Build history of the part. All positions in model axes, mm. Face numbers are marked on the shaded views. A direction names the side the tool comes from. Give positions to 0.01 mm unless a question says otherwise; leave off trailing zeros. Loops run counter-clockwise (first coordinate to the right, second up) from the corner with the lowest first, then second, coordinate; pieces in that order, holes last. Notation, with made-up numbers: (58, 81) -> (102, 81) arc R15 ccw to (102, 86) -> close; hole circle Ø10 at (8.5, 45). An arc over 180 degrees is marked (long way). Answer as a JSON object with one key per item and string values. Group by question number.
Q1. Band-saw the part on A-A, the plane y = 7.75. Write the cut outline in (x, z), plus the area to 3 significant figures.
Q2. Band-saw the part on B-B, the plane x = 16.25. Write the cut outline in (y, z), plus the area to 3 significant figures.
Q3. Band-saw the part on D-D, the plane z = 2.2. Write the cut outline in (x, y), plus the area to 3 significant figures.
Q4. Wall check: probe 1 along X at (y, z) = (15.75, 3.25); probe 2 along Y at (x, z) = (12, 1.85); probe 3 along X at (y, z) = (17.5, 0.4). Give the ranges that are in metal, low to high. Write a range as from..to.
Q5. Tool access for the marked faces 1 and 2: list every direction of +Z, -Z, +X, -X, +Y, -Y with a clear straight run to the whole face (end or side of a thin tool).
Q6. Band-saw the part on C-C, the plane y = 15.5. Write the cut outline in (x, z).
Q7. Drop flat-ended pins along their axis: pin 1 (5 mm diameter, centred on x = 15.52, y = 15.79, fed in from +Z); pin 2 (4 mm diameter, centred on x = 5.77, y = 15.79, fed in from +Z). Give the stop position or say it passes through.
Q8. Two-plate mould, pull along X, no slides. Class the marked faces 3, 4, 5 and 6: pulls with the +X half, pulls with the -X half, needs draft (parallel to the pull), parting line crosses it, or undercut.
from build123d import *

# Parameters (mm, degrees)
ESQUISSE1_W        = 21.281999849
ESQUISSE1_H        = 19.97412287
ESQUISSE1_R        = 2.13
ESQUISSE1_W_2      = 4
ESQUISSE1_H_2      = 7
BOSS_EXTRU_1_DEPTH = 4
CONG_1_R           = 2


with BuildPart() as part:
    # Esquisse1 → Boss.-Extru.1 (new body)
    with BuildSketch(Plane.XY):
        with Locations((10.640999925, 9.987061435)):
            Rectangle(ESQUISSE1_W, ESQUISSE1_H)
        with Locations((5.765999924, 15.79412287)):
            Circle(ESQUISSE1_R, mode=Mode.SUBTRACT)
        with Locations((15.515999924, 15.79412287)):
            Circle(ESQUISSE1_R, mode=Mode.SUBTRACT)
        with Locations((10.640999924, 5.79412287)):
            Rectangle(ESQUISSE1_W_2, ESQUISSE1_H_2, mode=Mode.SUBTRACT)
    extrude(amount=BOSS_EXTRU_1_DEPTH)

    # Congé1
    cong_1_edges = [part.edges().sort_by_distance(p)[0] for p in [
        (0, 19.97412287, 2),
        (21.281999849, 19.97412287, 2),
        (21.281999849, 0, 2),
        (0, 0, 2),
    ]]
    fillet(cong_1_edges, radius=CONG_1_R)


solid = part.part
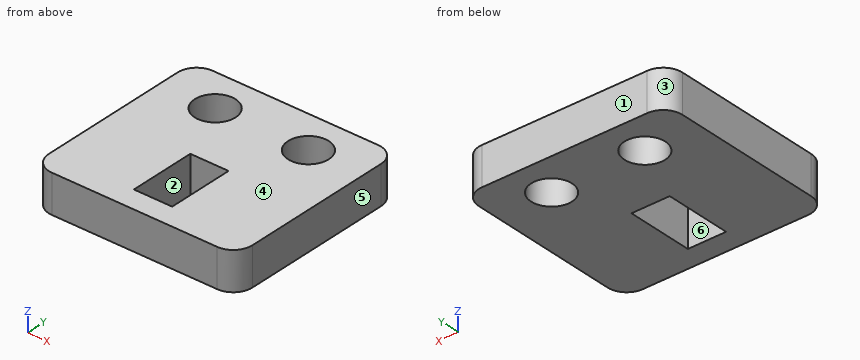
Worked answers:
{
 "1": {"outline": "(0, 0) -> (8.64, 0) -> (8.64, 4) -> (0, 4) -> close; (12.64, 0) -> (21.28, 0) -> (21.28, 4) -> (12.64, 4) -> close", "area": "69.1 mm2"},
 "2": {"outline": "(0, 0) -> (13.79, 0) -> (13.79, 4) -> (0, 4) -> close; (17.79, 0) -> (19.97, 0) -> (19.97, 4) -> (17.79, 4) -> close", "area": "63.9 mm2"},
 "3": {"outline": "(0, 2) arc R2 ccw to (2, 0) -> (19.28, 0) arc R2 ccw to (21.28, 2) -> (21.28, 17.97) arc R2 ccw to (19.28, 19.97) -> (2, 19.97) arc R2 ccw to (0, 17.97) -> close; hole circle Ø4.26 at (5.77, 15.79); hole (8.64, 2.29) -> (12.64, 2.29) -> (12.64, 9.29) -> (8.64, 9.29) -> close; hole circle Ø4.26 at (15.52, 15.79)", "area": "365 mm2"},
 "4": {"probe 1": "0..3.64, 7.9..13.39, 17.65..21.28", "probe 2": "0..2.29, 9.29..19.97", "probe 3": "0..4.49, 7.04..14.24, 16.79..21.28"},
 "5": {"face 1": "+Z, -Z, +X, -X, +Y", "face 2": "+Z, -Z"},
 "6": {"outline": "(0, 0) -> (3.66, 0) -> (3.66, 4) -> (0, 4) -> close; (7.88, 0) -> (13.41, 0) -> (13.41, 4) -> (7.88, 4) -> close; (17.63, 0) -> (21.28, 0) -> (21.28, 4) -> (17.63, 4) -> close"},
 "7": {"pin 1": "z = 4", "pin 2": "through"},
 "8": {"face 3": "pulls with the -X half", "face 4": "needs draft", "face 5": "pulls with the +X half", "face 6": "undercut"}
}
